The listing builds one solid part. Answer for the finished solid, in the listing's coordinates (mm). A direction names the side the tool comes from. Give positions to 0.01 mm unless a question says otherwise; leave off trailing zeros. Write each loop counter-clockwise with the first axis right and the second up, starting at its lowest first coordinate (ties: lowest second). Pieces come first, ordered by that corner, then holes. Notation, with made-up numbers: (23, -23) -> (50, -23) arc R15 cw to (50, 3) -> close; hole circle Ø8 at (56, -30). An arc over 180 degrees is marked (long way). One line per question, with ' | ' between items.
Autodesk Inventor part; units mm, degrees
ref_plane "Work Plane1" through (44.5423, 0, 0) normal (0, 0, -1) x (-1, 0, 0)
ref_plane "YZ Plane" through (0, 0, 0) normal (1, 0, 0) x (0, 1, 0)
ref_plane "XZ Plane" through (0, 0, 0) normal (0, 1, 0) x (-1, 0, 0)
sketch "Sketch1" plane through (0, 0, 0) normal (0, 0, 1) x (1, 0, 0)
  line L0 (-3.2274, 0) -> (16.8712, 0)
  line L1 (5.5129, 10.5) -> (4.0032, 13.7375)
  line L2 (5.5129, 10.5) -> (14, 10.5) construction
  line L3 (14, 10.5) -> (14, 0) construction
  arc A0 (4.0032, 13.7375) -> (0, 12.85) centre (2.1, 12.85) ccw
  line L4 (5.5129, 10.5) -> (5.5129, 0)
  line L5 (0, -3.0688) -> (0, 18.4128)
  point P0 (0, 0)
  dimension "d2" = 21
  dimension "d4" = 29.9
  dimension "d5" = 2.1
  dimension "d15" = 14
  dimension "d16" = 25
revolve "Ring" add sketch "Sketch1" angle 360 about axis through (-10, 0, 0) along (1, 0, 0)
sketch "Sketch2" plane through (0, 0, 0) normal (-1, 0, 0) x (0, 0, 1)
  circle A0 centre (0, 0) radius 4.9
  line L0 (-10.5, -6.0622) -> (-10.5, 6.0622)
  line L1 (-10.5, 6.0622) -> (0, 12.1244)
  line L2 (0, 12.1244) -> (10.5, 6.0622)
  line L3 (10.5, 6.0622) -> (10.5, -6.0622)
  line L4 (10.5, -6.0622) -> (0, -12.1244)
  line L5 (0, -12.1244) -> (-10.5, -6.0622)
  circle A1 centre (0, 0) radius 12.85
  dimension "d6" = 24.2487
extrude "Body" add sketch "Sketch2" against normal blind 14 contours A0 | L0 L1 L2 L3 L4 L5
sketch "Sketch3" plane through (0, 0, 0) normal (0, 0, 1) x (1, 0, 0)
  line L0 (4.7555, 12.1244) -> (14, 12.1244)
  line L1 (14, 6.0622) -> (14, 12.1244)
  line L2 (0, -12.85) -> (0, 12.85)
  line L3 (-2.8, 0) -> (16.8, 0)
  line L4 (13.0622, 12.1244) -> (14, 10.5)
  dimension "d10" = 30
  dimension "d11" = 21
revolve "Chamfer1" cut sketch "Sketch3" angle 360 about axis through (-10, 0, 0) along (1, 0, 0)
sketch "Sketch4" plane through (0, 0, 0) normal (-1, 0, 0) x (0, 0, 1)
  circle A0 centre (0, 0) radius 12.85
hole "Thread" at (0, 0, 0) direction (1, 0, 0) diameter 11.835 end through all
chamfer "Chamfer2" distance 1.0825 angle 30 1 edges at (0, 0, -5.9175) measured on face at (0, 10.4003, -1.2628)
ref_plane "Work Plane1" through (44.5423, 0, 0) normal (0, 0, -1) x (-1, 0, 0)
chamfer "Chamfer3" distance 1.0825 angle 45 1 edges at (14, 0, -5.9175)
equation "\"d6\" = 1.1547 * SW"
equation "\"d7\" = KOH"
equation "\"d12\" = -0.5 * GD1 + 0.5 * NND"
equation "\"d46\" = -0.5 * GD1 + 0.5 * NND"
equation "\"d51\" = -0.5 * GD1 + 0.5 * NND"
equation "\"d2\" = SW"
equation "\"d4\" = LADI"
equation "\"d5\" = PHH"
equation "\"d15\" = KOH"
equation "\"d16\" = KEWI"
equation "\"d10\" = ANG1"
equation "\"d11\" = SW0"
equation "\"ANG1\" = 30deg"
equation "\"KEWI\" = 25deg"
equation "\"NND\" = 14"
equation "\"LADI\" = 29.9"
equation "\"SW\" = 21"
equation "\"PHH\" = 2.1"
equation "\"KOH\" = NND"
equation "\"SW0\" = 21"
equation "\"d1\" = LADI"
equation "\"d3\" = PHH"
equation "\"GUL\" = 0.541266 * PTC"
equation "\"RR\" = PHH"
equation "\"THREADDIA\" = 14"
equation "\"TOA\" = 30deg"
equation "\"PTC\" = 2"
equation "\"GAL\" = 0.541266 * PTC"
equation "\"E0\" = 1.155 * SW"
properties part number "ISO 4161 - M14" material "Stainless Steel"
Item 1: A tool of negligible diameter and unlimited length cuts with its end or side. For faces 1 (the face through (9.313, -9.136, -5.176)), 2 (the face through (13.839, 10.776, 0.237)), 3 (the face through (9.313, -9.051, 5.324)), from which of +Z, -Z, +X, -X, +Y, -Y can it reach the whole face along a straight path? Write none if from no direction.
Answers below:
face 1: -Z, +X, -Y | face 2: +X, +Y | face 3: +Z, +X, -Y
Item 2: Find section A-A (x = 10.5). Write down the section's boundary in (y, z) (1 decimal), then the cut area to 3 significant figures.
Answers below:
outline: (-12.1, 0) -> (-6.1, -10.5) -> (6.1, -10.5) -> (12.1, 0) -> (6.1, 10.5) -> (-6.1, 10.5) -> close; hole circle Ø11.8 at (0, 0) | area: 272 mm²
Item 3: Consider line 1 (Y direction, x = 5.5, z = 0); line 2 (Z direction, x = 6.5, y = 0); line 3 (Z direction, x = 5, y = 3). Determine where each line is inside the solid, lowest interval first. Write a range as [from, to].
Answers below:
line 1: [-12.12, -5.92], [5.92, 12.12] | line 2: [-10.5, -5.92], [5.92, 10.5] | line 3: [-11.21, -5.1], [5.1, 11.21]
Item 4: Determine the mould class of faces 4 (the face through (6.857, -5.867, -0.77)), 5 (the face through (9.313, 9.136, 5.176)), 6 (the face through (13.839, -10.776, -0.237)), 7 (the face through (9.313, 9.051, -5.324)) for opening direction Z: pulls with the +Z half, pulls with the -Z half, needs draft (parallel to the pull), parting line crosses it, or undercut.
Answers below:
face 4: undercut | face 5: pulls with the +Z half | face 6: parting line crosses it | face 7: pulls with the -Z half
Item 5: Flat-ended cylindrical pins translate along their axes: pin 1 (15.5 mm diameter, centred on y = 0, z = 0, fed in from +X); pin 2 (1 mm diameter, centred on x = 9.5, z = 1, fed in from -Y); pin 3 (4.5 mm diameter, centred on x = 8, y = -2, fed in from +Z); pin 4 (3 mm diameter, centred on x = 8.5, y = -3, fed in from -Z). Find the tip coordinate at first contact, or state that the pin passes through.
Answers below:
pin 1: x = 14 | pin 2: y = -11.84 | pin 3: z = 10.5 | pin 4: z = -10.5
